Check sheet for the modelled part. Datum: model origin and axes. Units: mm. Face numbers are marked on the shaded views. A direction names the side the tool comes from. Coordinates: 2 decimals unless noted, no trailing zeros. Order: outer loops, then holes, each group sorted by start corner. A loop starts at its lowest first (then second) coordinate and runs counter-clockwise, first axis right, second up. Notation, with made-up numbers: (36.5, 6) -> (51.5, 6) arc R19 ccw to (51.5, 33) -> close; hole circle Ø9 at (0.25, 31.25). An arc over 180 degrees is marked (long way). Put each result on its own line as item: value. Start each with the question number.
```python
from build123d import *

# Parameters (mm, degrees)
BOSS_EXTRUDE1_DEPTH = 30
SKETCH3_R           = 1.55
CUT_EXTRUDE1_DEPTH  = 22
CUT_EXTRUDE2_START  = -30
SKETCH5_R           = 1.55
CUT_EXTRUDE2_DEPTH  = 30
SKETCH6_R           = 3
CUT_EXTRUDE3_DEPTH  = 5
SKETCH7_R           = 8
CUT_EXTRUDE10_DEPTH = 5
SKETCH8_R           = 5
SKETCH8_R_2         = 1.05
CUT_EXTRUDE7_DEPTH  = 8
SKETCH9_R           = 2.2
CUT_EXTRUDE8_DEPTH  = 2.5


with BuildPart() as part:
    # Sketch1 → Boss-Extrude1 (new body)
    with BuildSketch(Plane.XY):
        with BuildLine():
            Line((-1.5, 49.363448016), (43.5, 23.382685902))
            ThreePointArc((43.5, 23.382685902), (57, 0), (43.5, -23.382685902))
            Line((43.5, -23.382685902), (-1.5, -49.363448016))
            ThreePointArc((-1.5, -49.363448016), (-87, 0), (-1.5, 49.363448016))
        make_face()
    extrude(amount=BOSS_EXTRUDE1_DEPTH)

    # Sketch3 → Cut-Extrude1 (cut)
    with BuildSketch(Plane.XY.offset(30)):
        with Locations((50.449984706, 0.025940866)):
            Circle(SKETCH3_R)
        with Locations((-80.45, 0)):
            Circle(SKETCH3_R)
        with Locations((-65.673537111, 35.673537111)):
            Circle(SKETCH3_R)
        with Locations((-65.673537111, -35.673537111)):
            Circle(SKETCH3_R)
        with Locations((7.233447448, 36.661458689)):
            Circle(SKETCH3_R)
        with Locations((7.291641994, -36.724302618)):
            Circle(SKETCH3_R)
        with BuildLine():
            Line((50.449984706, 3.525940866), (53.739581736, 3.525940866))
            ThreePointArc((53.739581736, 3.525940866), (49.844264614, 13.498339229), (42, 20.784609691))
            Line((42, 20.784609691), (12.081289905, 38.058185018))
            Line((12.081289905, 38.058185018), (10.268372938, 34.918120721))
            ThreePointArc((10.268372938, 34.918120721), (5.49010948, 33.626533199), (4.198521958, 38.404796657))
            Line((4.198521958, 38.404796657), (6.019126703, 41.558176575))
            Line((6.019126703, 41.558176575), (-3, 46.765371804))
            ThreePointArc((-3, 46.765371804), (-35.308766962, 53.738412643), (-65.628603797, 40.578351266))
            Line((-65.628603797, 40.578351266), (-63.198663377, 38.148410845))
            ThreePointArc((-63.198663377, 38.148410845), (-63.198663377, 33.198663377), (-68.148410845, 33.198663377))
            Line((-68.148410845, 33.198663377), (-70.578351266, 35.628603797))
            ThreePointArc((-70.578351266, 35.628603797), (-79.889494756, 20.664905348), (-83.886454699, 3.5))
            Line((-83.886454699, 3.5), (-80.45, 3.5))
            ThreePointArc((-80.45, 3.5), (-76.95, 0), (-80.45, -3.5))
            Line((-80.45, -3.5), (-83.886454699, -3.5))
            ThreePointArc((-83.886454699, -3.5), (-79.889494756, -20.664905348), (-70.578351266, -35.628603797))
            Line((-70.578351266, -35.628603797), (-68.148410845, -33.198663377))
            ThreePointArc((-68.148410845, -33.198663377), (-63.198663377, -33.198663377), (-63.198663377, -38.148410845))
            Line((-63.198663377, -38.148410845), (-65.628603797, -40.578351266))
            ThreePointArc((-65.628603797, -40.578351266), (-35.308766962, -53.738412643), (-3, -46.765371804))
            Line((-3, -46.765371804), (6.035553081, -41.548692801))
            Line((6.035553081, -41.548692801), (4.260553081, -38.474302618))
            ThreePointArc((4.260553081, -38.474302618), (5.541641994, -33.693213705), (10.322730907, -34.974302618))
            Line((10.322730907, -34.974302618), (12.097730907, -38.048692801))
            Line((12.097730907, -38.048692801), (42, -20.784609691))
            ThreePointArc((42, -20.784609691), (49.859000377, -13.476650327), (53.747229589, -3.474059134))
            Line((53.747229589, -3.474059134), (50.449984706, -3.474059134))
            ThreePointArc((50.449984706, -3.474059134), (46.949984706, 0.025940866), (50.449984706, 3.525940866))
        make_face()
    extrude(amount=-CUT_EXTRUDE1_DEPTH, mode=Mode.SUBTRACT)

    # Sketch5 → Cut-Extrude2 (cut)
    with BuildSketch(Plane(origin=(0, 0, 0), x_dir=(-1, 0, 0), z_dir=(0, 0, -1)).offset(CUT_EXTRUDE2_START)):
        with Locations(Location((65.673537111, 35.673537111, 0), (0, 0, 180))):
            Circle(SKETCH5_R)
        with Locations(Location((80.45, 0, 0), (0, 0, 180))):
            Circle(SKETCH5_R)
        with Locations(Location((-7.233447448, 36.661458689, 0), (0, 0, 180))):
            Circle(SKETCH5_R)
        with Locations(Location((-50.449984706, 0.025940866, 0), (0, 0, 180))):
            Circle(SKETCH5_R)
        with Locations(Location((-7.291641994, -36.724302618, 0), (0, 0, 180))):
            Circle(SKETCH5_R)
        with Locations(Location((65.673537111, -35.673537111, 0), (0, 0, 180))):
            Circle(SKETCH5_R)
    extrude(amount=CUT_EXTRUDE2_DEPTH, mode=Mode.SUBTRACT)

    # Sketch6 → Cut-Extrude3 (cut)
    with BuildSketch(Plane(origin=(0, 0, 0), x_dir=(-1, 0, 0), z_dir=(0, 0, -1))):
        with Locations((-50.449984706, 0.025940866)):
            Circle(SKETCH6_R)
        with Locations((-7.291641994, -36.724302618)):
            Circle(SKETCH6_R)
        with Locations((65.673537111, -35.673537111)):
            Circle(SKETCH6_R)
        with Locations((80.45, 0)):
            Circle(SKETCH6_R)
        with Locations((65.673537111, 35.673537111)):
            Circle(SKETCH6_R)
        with Locations((-7.233447448, 36.661458689)):
            Circle(SKETCH6_R)
    extrude(amount=-CUT_EXTRUDE3_DEPTH, mode=Mode.SUBTRACT)

    # Sketch7 → Cut-Extrude10 (cut)
    with BuildSketch(Plane.XY.offset(8)):
        with Locations((-29.795862437, 0)):
            Circle(SKETCH7_R)
        with Locations((30, 0)):
            Circle(SKETCH7_R)
    extrude(amount=-CUT_EXTRUDE10_DEPTH, mode=Mode.SUBTRACT)

    # Sketch8 → Cut-Extrude7 (cut)
    with BuildSketch(Plane.XY.offset(8)):
        with Locations((-30, 0)):
            Circle(SKETCH8_R)
        with Locations((-38.980256121, 8.980256121)):
            Circle(SKETCH8_R_2)
        with Locations((-21.019743879, 8.980256121)):
            Circle(SKETCH8_R_2)
        with Locations((-21.019743879, -8.980256121)):
            Circle(SKETCH8_R_2)
        with Locations((-38.980256121, -8.980256121)):
            Circle(SKETCH8_R_2)
    extrude(amount=-CUT_EXTRUDE7_DEPTH, mode=Mode.SUBTRACT)

    # Sketch9 → Cut-Extrude8 (cut)
    with BuildSketch(Plane.XY.offset(8)):
        with Locations((-38.980256121, 8.980256121)):
            Circle(SKETCH9_R)
        with Locations((-21.019743879, 8.980256121)):
            Circle(SKETCH9_R)
        with Locations((-21.019743879, -8.980256121)):
            Circle(SKETCH9_R)
        with Locations((-38.980256121, -8.980256121)):
            Circle(SKETCH9_R)
    extrude(amount=-CUT_EXTRUDE8_DEPTH, mode=Mode.SUBTRACT)


solid = part.part
```
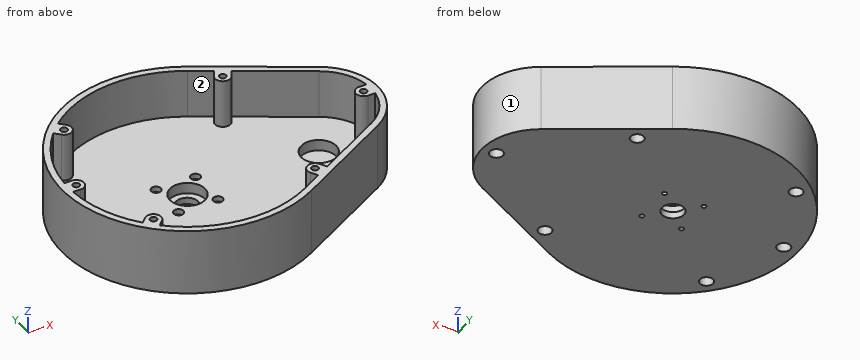
1) Sectioned sample at C-C (y = 25.5). Record the boundary of the cut face in (x, z).
2) Access from +Z, -Z, +X, -X, +Y, -Y to the whole of each face (thin tool, end or side, straight path). Record for the marked faces 1 and 2.
3) Sectioned sample at A-A (x = -30). Record the boundary of the cut face in (y, z), plus the area to 3 significant figures.
4) Gauge pin test, flat ends, axial feed: pin 1 (1.5 mm diameter, centred on x = -37.5, y = 18, fed in from +Z); pin 2 (3.5 mm diameter, centred on x = -38.98, y = 8.98, fed in from +Z); pin 3 (10 mm diameter, centred on x = -58.5, z = 12.5, fed in from +Y); pin 4 (1.9 mm diameter, centred on x = -80.45, y = 0, fed in from -Z). Record the tip position at first contact, or that the pin passes through.
5) Scan lines: line 1 along Y through (x, z) = (-29, 6); line 2 along Y through (x, z) = (-30, 1); line 3 along Z through (x, y) = (-26, -43.5). Record each from-to range of solid material in increasing order. Write a range as [from, to].
6) Sectioned sample at D-D (z = 15.75). State how many separate pieces and enclosed holes the cut face has, plus the area to 3 significant figures.
7) Sectioned sample at B-B (x = -54). Record the boundary of the cut face in (y, z).
Entries:
1. outline: (-80.98, 0) -> (39.83, 0) -> (39.83, 30) -> (33.83, 30) -> (33.83, 8) -> (-77.6, 8) -> (-77.6, 30) -> (-80.98, 30) -> close
2. face 1: +Z, -Z, +X
2. face 2: +Z
3. outline: (-57, 0) -> (-5, 0) -> (-5, 3) -> (-8, 3) -> (-8, 8) -> (-54, 8) -> (-54, 30) -> (-57, 30) -> close; (5, 0) -> (57, 0) -> (57, 30) -> (54, 30) -> (54, 8) -> (8, 8) -> (8, 3) -> (5, 3) -> close
3. area: 934 mm2
4. pin 1: stops at z = 8
4. pin 2: stops at z = 5.5
4. pin 3: stops at y = 51.93
4. pin 4: passes through
5. line 1: y = [-56.99, -7.96], [7.96, 56.99]
5. line 2: y = [-57, -5], [5, 57]
5. line 3: z = [0, 8]
6. separate pieces: 1
6. enclosed holes: 7
6. area: 1,390 mm2
7. outline: (-51.7, 0) -> (51.7, 0) -> (51.7, 30) -> (48.37, 30) -> (48.37, 8) -> (-48.37, 8) -> (-48.37, 30) -> (-51.7, 30) -> close
